Can you work these out from the model? Positions are in its coordinate system, mm. A direction names the side the tool comes from. Coordinates: 2 decimals unless noted, no trailing zeros. Order: outer loops, then holes, each group sorted by start corner. A loop starts at its lowest first (then second) coordinate and runs counter-clockwise, first axis right, second up. Notation, with made-up numbers: (44.25, 79.5) -> (65.25, 79.5) arc R21 cw to (65.25, 99.5) -> close; hole circle Ø8 at (-16.5, 25). An arc over 180 degrees is marked (long way). Answer as a JSON object with one key per item and string values. Group by question number.
(1) Which directions (+Z, -Z, +X, -X, +Y, -Y) give clear straight access to the entire face, cutting with the end or side of a thin tool? Please do faces 5 (the cylindrical face through (7.753, 2.643, 2.521)), 6 (the cylindrical face through (17.25, -8.42, 2.03)).
(2) For pin 1 (4 mm diameter, centred on x = 11, y = 2.5, fed in from +Z), with a flat end and sliding along its axis, tell me the tip position at first contact or that it passes through.
(3) I want a section at D-D, the plane z = 3.1. List the corners of the cut face in (x, y) for me, plus the area to 3 significant figures.
(4) I want a section at C-C, the plane x = 19. List the corners of the cut face in (y, z) for me, plus the area to 3 significant figures.
(5) I want a section at B-B, the plane z = 0.5. List the corners of the cut face in (x, y) for me, plus the area to 3 significant figures.
(6) I need wall thicknesses on line 1 (Y direction, x = -19, z = 1.55); line 2 (X direction, y = -9, z = 2.9); line 3 (X direction, y = 4, z = 3.2). Which ranges of each line are inside material? Lowest first, please.
(7) If we mould it in two halves opening along X, with no side actions, what happens to faces 1 (the cylindrical face through (18.772, 15.235, 2.028)), 2 (the cylindrical face through (-14.247, 2.643, 2.521)), 3 (the flat face through (22.5, 0, 2)), 4 (the flat face through (0, 17.5, 2))? For each: pulls with the +X half, pulls with the -X half, needs draft (parallel to the pull), parting line crosses it, or undercut.
(8) I want a section at A-A, the plane y = -8.5. List the corners of the cut face in (x, z) for me, plus the area to 3 significant figures.
from build123d import *

# Parameters (mm, degrees)
SKETCH_1_W          = 45
SKETCH_1_H          = 35
EXTRUDE_1_DEPTH     = 4
SKETCH_2_R          = 1.75
CUT_EXTRUDE_1_DEPTH = 5
SKETCH_3_R          = 3.25
CUT_EXTRUDE_2_DEPTH = 3


with BuildPart() as part:
    # ｽｹｯﾁ1 → ﾎﾞｽ - 押し出し1 (new body)
    with BuildSketch(Plane.XY):
        Rectangle(SKETCH_1_W, SKETCH_1_H)
    extrude(amount=EXTRUDE_1_DEPTH)

    # ｽｹｯﾁ2 → ｶｯﾄ - 押し出し1 (cut, through all)
    with BuildSketch(Plane.XY.offset(4)):
        with Locations((-19, 13.5)):
            Circle(SKETCH_2_R)
        with Locations((-19, -8.5)):
            Circle(SKETCH_2_R)
        with Locations((19, 13.5)):
            Circle(SKETCH_2_R)
        with Locations((19, -8.5)):
            Circle(SKETCH_2_R)
        with Locations((-11, 2.5)):
            Circle(SKETCH_2_R)
        with Locations((11, 2.5)):
            Circle(SKETCH_2_R)
    extrude(amount=-CUT_EXTRUDE_1_DEPTH, mode=Mode.SUBTRACT)

    # ｽｹｯﾁ3 → ｶｯﾄ - 押し出し2 (cut)
    with BuildSketch(Plane.XY.offset(4)):
        with Locations((-11, 2.5)):
            Circle(SKETCH_3_R)
        with Locations((11, 2.5)):
            Circle(SKETCH_3_R)
    extrude(amount=-CUT_EXTRUDE_2_DEPTH, mode=Mode.SUBTRACT)


solid = part.part
Computed values:
{
 "1": {"face 5": "+Z", "face 6": "+Z, -Z"},
 "2": {"pin 1": "stops at z = 1"},
 "3": {"outline": "(-22.5, -17.5) -> (22.5, -17.5) -> (22.5, 17.5) -> (-22.5, 17.5) -> close; hole circle Ø3.5 at (-19, -8.5); hole circle Ø3.5 at (-19, 13.5); hole circle Ø6.5 at (-11, 2.5); hole circle Ø6.5 at (11, 2.5); hole circle Ø3.5 at (19, -8.5); hole circle Ø3.5 at (19, 13.5)", "area": "1,470 mm2"},
 "4": {"outline": "(-17.5, 0) -> (-10.25, 0) -> (-10.25, 4) -> (-17.5, 4) -> close; (-6.75, 0) -> (11.75, 0) -> (11.75, 4) -> (-6.75, 4) -> close; (15.25, 0) -> (17.5, 0) -> (17.5, 4) -> (15.25, 4) -> close", "area": "112 mm2"},
 "5": {"outline": "(-22.5, -17.5) -> (22.5, -17.5) -> (22.5, 17.5) -> (-22.5, 17.5) -> close; hole circle Ø3.5 at (-19, -8.5); hole circle Ø3.5 at (-19, 13.5); hole circle Ø3.5 at (-11, 2.5); hole circle Ø3.5 at (11, 2.5); hole circle Ø3.5 at (19, -8.5); hole circle Ø3.5 at (19, 13.5)", "area": "1,520 mm2"},
 "6": {"line 1": "y = -17.5 to -10.25, -6.75 to 11.75, 15.25 to 17.5", "line 2": "x = -22.5 to -20.68, -17.32 to 17.32, 20.68 to 22.5", "line 3": "x = -22.5 to -13.88, -8.12 to 8.12, 13.88 to 22.5"},
 "7": {"face 1": "undercut", "face 2": "undercut", "face 3": "pulls with the +X half", "face 4": "needs draft"},
 "8": {"outline": "(-22.5, 0) -> (-20.75, 0) -> (-20.75, 4) -> (-22.5, 4) -> close; (-17.25, 0) -> (17.25, 0) -> (17.25, 4) -> (-17.25, 4) -> close; (20.75, 0) -> (22.5, 0) -> (22.5, 4) -> (20.75, 4) -> close", "area": "152 mm2"}
}
